Autodesk Inventor part; units mm, degrees
ref_plane "YZ Plane" through (0, 0, 0) normal (1, 0, 0) x (0, 1, 0)
ref_plane "XZ Plane" through (0, 0, 0) normal (0, 1, 0) x (-1, 0, 0)
ref_plane "XY Plane" through (0, 0, 0) normal (0, 0, 1) x (1, 0, 0)
sketch "Sketch1" plane through (0, 0, 0) normal (0, 0, 1) x (1, 0, 0)
  line L0 (0, 110.8966) -> (0, -110.8966) construction
  line L1 (-205.6207, 0) -> (205.6207, 0) construction
  line L2 (-67, 75) -> (-220, 75)
  line L3 (-220, 75) -> (-158.9525, 32.2541)
  line L4 (-140, 0) -> (-100, 0)
  arc A0 (-140, 0) -> (-158.9525, 32.2541) centre (-184.7635, -4.6077) ccw
  arc A1 (0, -100) -> (-100, 0) centre (-100, -100) ccw
  arc A2 (0, 55) -> (-12, 52.4955) centre (0, 25) ccw
  line L5 (-12, 52.4955) -> (-16.3057, 65)
  line L6 (-16.3057, 65) -> (-19.1435, 38)
  arc A3 (-67, 75) -> (-19.1435, 38) centre (-25.2476, 79.5541) ccw
  line L7 (205.6207, 0) -> (-205.6207, 0) construction
  line L8 (67, 75) -> (220, 75)
  line L9 (220, 75) -> (158.9525, 32.2541)
  line L10 (140, 0) -> (100, 0)
  arc A4 (158.9525, 32.2541) -> (140, 0) centre (184.7635, -4.6077) ccw
  arc A5 (100, 0) -> (0, -100) centre (100, -100) ccw
  arc A6 (12, 52.4955) -> (0, 55) centre (0, 25) ccw
  line L11 (12, 52.4955) -> (16.3057, 65)
  line L12 (16.3057, 65) -> (19.1435, 38)
  arc A7 (19.1435, 38) -> (67, 75) centre (25.2476, 79.5541) ccw
  point P0 (0, 0)
  point P1 (0, 0)
  dimension "d1" = 67
  dimension "d2" = 220
  dimension "d3" = 35
  dimension "d4" = 45
  dimension "d5" = 140
  dimension "d7" = 75
  dimension "d8" = 100
  dimension "d9" = 100
  dimension "d10" = 30
  dimension "d11" = 50
  dimension "d12" = 12
  dimension "d13" = 10
  dimension "d14" = 37
  dimension "d15" = 25
  dimension "d21" = 42
  dimension "d23" = 84
extrude "Extrusion1" add sketch "Sketch1" along normal blind 25
properties part number "Batarang"
Check sheet for the modelled part. Datum: model origin and axes. Units: mm. A direction names the side the tool comes from. Coordinates: 2 decimals unless noted, no trailing zeros. Loops run counter-clockwise (first coordinate to the right, second up) from the corner with the lowest first, then second, coordinate; pieces in that order, holes last.
1) Sectioned sample at B-B (z = 15.75). Record the boundary of the cut face in (x, y), and give its area (3 significant figures).
2) Sectioned sample at D-D (y = -46). Record the boundary of the cut face in (x, z), and give its area (3 significant figures).
3) Release check for a two-part mould opening along X. For faces 4 (the face through (-3, 28, 25)), 5 (the face through (-30.071, -28.516, 12.325)), 6 (the face through (189.904, 53.926, 12.325)), 7 (the face through (-14.123, 58.66, 12.325)) record: released by +X, released by -X, zero draft, split by the parting line, or undercut.
4) Gauge pin test, flat ends, axial feed: pin 1 (8 mm diameter, centred on x = 55.5, z = 7, fed in from -Y); pin 2 (7.5 mm diameter, centred on x = 116.5, z = 16, fed in from -Y); pin 3 (5 mm diameter, centred on y = 46, z = 10.5, fed in from +X); pin 4 (1 mm diameter, centred on x = -6, y = -37, fed in from -Z). Record the tip position at first contact, or that the pin passes through.
5) Material ranges on probe 1 along X at (y, z) = (52, 8); probe 2 along X at (y, z) = (-26.5, 3.25); probe 3 along X at (y, z) = (-90.5, 4), recorded low to high.
6) Sectioned sample at A-A (y = 48). Record the boundary of the cut face in (x, z).
7) Sectioned sample at C-C (x = 180). Record the boundary of the cut face in (y, z), and give its area (3 significant figures).
8) Access from +Z, -Z, +X, -X, +Y, -Y to the whole of each face (thin tool, end or side, straight path). Record for faces 1 (the face through (-17.705, 51.689, 12.325)), 2 (the face through (-146.1, 18.42, 12.32)), 3 (the face through (120, 0, 12)).
Check sheet entries:
1. outline: (-220, 75) - (-158.95, 32.25) arc R45 cw to (-140, 0) - (-100, 0) arc R100 cw to (0, -100) arc R100 cw to (100, 0) - (140, 0) arc R45 cw to (158.95, 32.25) - (220, 75) - (67, 75) arc R42 cw to (19.14, 38) - (16.31, 65) - (12, 52.5) arc R30 ccw to (0, 55) arc R30 ccw to (-12, 52.5) - (-16.31, 65) - (-19.14, 38) arc R42 cw to (-67, 75) - close
1. area: 26,300 mm2
2. outline: (-15.83, 0) - (15.83, 0) - (15.83, 25) - (-15.83, 25) - close
2. area: 792 mm2
3. face 4: zero draft
3. face 5: released by -X
3. face 6: released by +X
3. face 7: undercut
4. pin 1: stops at y = -12.55
4. pin 2: stops at y = 0
4. pin 3: stops at x = 182.15
4. pin 4: stops at z = 0
5. probe 1: x = -187.15 to -56.95, -17.67 to 17.67, 56.95 to 187.15
5. probe 2: x = -32.19 to 32.19
5. probe 3: x = -0.45 to 0.45
6. outline: (-181.44, 0) - (-52.97, 0) - (-52.97, 25) - (-181.44, 25) - close; (-18.09, 0) - (18.09, 0) - (18.09, 25) - (-18.09, 25) - close; (52.97, 0) - (181.44, 0) - (181.44, 25) - (52.97, 25) - close
7. outline: (46.99, 0) - (75, 0) - (75, 25) - (46.99, 25) - close
7. area: 700 mm2
8. face 1: +Z, -Z, +Y
8. face 2: +Z, -Z, -X, -Y
8. face 3: +Z, -Z, +X, -Y
